```python
from build123d import *

# Parameters (mm, degrees)
BOSS_EXTRUDE1_DEPTH = 1.9
SKETCH2_W           = 2
SKETCH2_H           = 5
BOSS_EXTRUDE2_DEPTH = 0.95


with BuildPart() as part:
    # Sketch1 → Boss-Extrude1 (new body)
    with BuildSketch(Plane(origin=(0, 0, 0), x_dir=(1, 0, 0), z_dir=(0, 1, 0))):
        with BuildLine():
            Line((172.5, 12.5), (0, 12.5))
            Line((0, 12.5), (0, 7.5))
            ThreePointArc((0, 7.5), (1.26826484, 7.391989197), (2.5, 7.071067812))
            ThreePointArc((2.5, 7.071067812), (12.5, 0), (2.5, -7.071067812))
            ThreePointArc((2.5, -7.071067812), (1.26826484, -7.391989197), (0, -7.5))
            Line((0, -7.5), (0, -12.5))
            Line((0, -12.5), (172.5, -12.5))
            ThreePointArc((172.5, -12.5), (182.747548784, 0), (172.5, 12.5))
        make_face()
        with BuildLine():
            ThreePointArc((47.5, -7.071067812), (37.5, 0), (47.5, 7.071067812))
            ThreePointArc((47.5, 7.071067812), (50, 7.5), (52.5, 7.071067812))
            ThreePointArc((52.5, 7.071067812), (55, 7.5), (57.5, 7.071067812))
            ThreePointArc((57.5, 7.071067812), (60, 7.5), (62.5, 7.071067812))
            ThreePointArc((62.5, 7.071067812), (65, 7.5), (67.5, 7.071067812))
            ThreePointArc((67.5, 7.071067812), (70, 7.5), (72.5, 7.071067812))
            ThreePointArc((72.5, 7.071067812), (75, 7.5), (77.5, 7.071067812))
            ThreePointArc((77.5, 7.071067812), (80, 7.5), (82.5, 7.071067812))
            ThreePointArc((82.5, 7.071067812), (85, 7.5), (87.5, 7.071067812))
            ThreePointArc((87.5, 7.071067812), (90, 7.5), (92.5, 7.071067812))
            ThreePointArc((92.5, 7.071067812), (95, 7.5), (97.5, 7.071067812))
            ThreePointArc((97.5, 7.071067812), (100, 7.5), (102.5, 7.071067812))
            ThreePointArc((102.5, 7.071067812), (105, 7.5), (107.5, 7.071067812))
            ThreePointArc((107.5, 7.071067812), (110, 7.5), (112.5, 7.071067812))
            ThreePointArc((112.5, 7.071067812), (122.5, 0), (112.5, -7.071067812))
            ThreePointArc((112.5, -7.071067812), (110, -7.5), (107.5, -7.071067812))
            ThreePointArc((107.5, -7.071067812), (105, -7.5), (102.5, -7.071067812))
            ThreePointArc((102.5, -7.071067812), (100, -7.5), (97.5, -7.071067812))
            ThreePointArc((97.5, -7.071067812), (95, -7.5), (92.5, -7.071067812))
            ThreePointArc((92.5, -7.071067812), (90, -7.5), (87.5, -7.071067812))
            ThreePointArc((87.5, -7.071067812), (85, -7.5), (82.5, -7.071067812))
            ThreePointArc((82.5, -7.071067812), (80, -7.5), (77.5, -7.071067812))
            ThreePointArc((77.5, -7.071067812), (75, -7.5), (72.5, -7.071067812))
            ThreePointArc((72.5, -7.071067812), (70, -7.5), (67.5, -7.071067812))
            ThreePointArc((67.5, -7.071067812), (65, -7.5), (62.5, -7.071067812))
            ThreePointArc((62.5, -7.071067812), (60, -7.5), (57.5, -7.071067812))
            ThreePointArc((57.5, -7.071067812), (55, -7.5), (52.5, -7.071067812))
            ThreePointArc((52.5, -7.071067812), (50, -7.5), (47.5, -7.071067812))
        make_face(mode=Mode.SUBTRACT)
        with BuildLine():
            ThreePointArc((137.5, 7.071067812), (140, 7.5), (142.5, 7.071067812))
            ThreePointArc((142.5, 7.071067812), (145, 7.5), (147.5, 7.071067812))
            ThreePointArc((147.5, 7.071067812), (150, 7.5), (152.5, 7.071067812))
            ThreePointArc((152.5, 7.071067812), (155, 7.5), (157.5, 7.071067812))
            ThreePointArc((157.5, 7.071067812), (160, 7.5), (162.5, 7.071067812))
            ThreePointArc((162.5, 7.071067812), (165, 7.5), (167.5, 7.071067812))
            ThreePointArc((167.5, 7.071067812), (177.5, 0), (167.5, -7.071067812))
            ThreePointArc((167.5, -7.071067812), (165, -7.5), (162.5, -7.071067812))
            ThreePointArc((162.5, -7.071067812), (160, -7.5), (157.5, -7.071067812))
            ThreePointArc((157.5, -7.071067812), (155, -7.5), (152.5, -7.071067812))
            ThreePointArc((152.5, -7.071067812), (150, -7.5), (147.5, -7.071067812))
            ThreePointArc((147.5, -7.071067812), (145, -7.5), (142.5, -7.071067812))
            ThreePointArc((142.5, -7.071067812), (140, -7.5), (137.5, -7.071067812))
            ThreePointArc((137.5, -7.071067812), (127.5, 0), (137.5, 7.071067812))
        make_face(mode=Mode.SUBTRACT)
    extrude(amount=BOSS_EXTRUDE1_DEPTH)

    # Sketch2 → Boss-Extrude2 (add)
    with BuildSketch(Plane(origin=(0, 0, 0), x_dir=(1, 0, 0), z_dir=(0, 1, 0))):
        with Locations((-1, 10)):
            Rectangle(SKETCH2_W, SKETCH2_H)
        with Locations((-1, -10)):
            Rectangle(SKETCH2_W, SKETCH2_H)
    extrude(amount=BOSS_EXTRUDE2_DEPTH)


solid = part.part
```
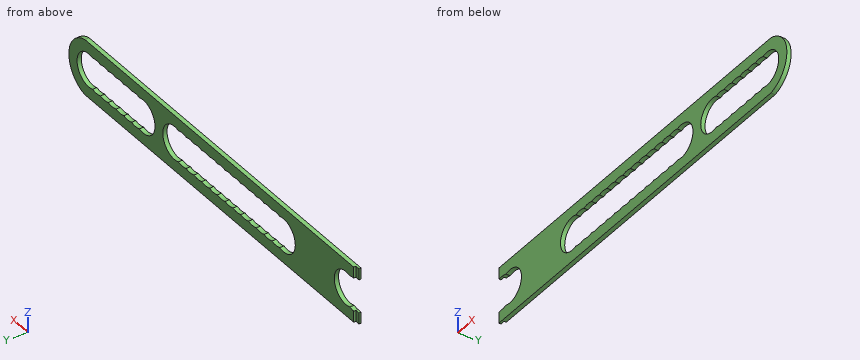
CAD build for the part. Positions are in the model's coordinates, mm. Coordinates: 2 decimals unless noted, no trailing zeros. Order: outer loops, then holes, each group sorted by start corner. A loop starts at its lowest first (then second) coordinate and runs counter-clockwise, first axis right, second up. Notation, with made-up numbers: (-21.75, -20.5) - (37.25, -20.5) arc R15 ccw to (37.25, -2.5) - close; hole circle Ø5 at (78, 38.5). An arc over 180 degrees is marked (long way). Answer in a Markdown table with one row per item.
1. Flat gauge pins, fed straight in: P1, Ø6, axis at x = 88, z = 2.5, coming from the +Y side; P2, Ø1.6, axis at x = -1, z = -9.5, coming from the +Y side. Where does each tip first touch, or does it go through?
Answer:
| item | result |
|---|---|
| P1 | through |
| P2 | y = 0.95 |
2. Slice it at D-D, the plane y = 0.6. Give the number of separate pieces and of enclosed holes in the cut face, then the cut area to 3 significant figures.
Answer:
| item | result |
|---|---|
| separate pieces | 1 |
| enclosed holes | 2 |
| area | 2,460 mm² |
3. Slice it at A-A, the plane z = 0. List the corners of the cut face in (x, y).
Answer:
| item | result |
|---|---|
| outline | (12.5, 0) - (37.5, 0) - (37.5, 1.9) - (12.5, 1.9) - close; (122.5, 0) - (127.5, 0) - (127.5, 1.9) - (122.5, 1.9) - close; (177.5, 0) - (182.75, 0) - (182.75, 1.9) - (177.5, 1.9) - close |
4. Slice it at B-B, the plane x = 115. List the corners of the cut face in (y, z).
Answer:
| item | result |
|---|---|
| outline | (0, -12.5) - (1.9, -12.5) - (1.9, -7.5) - (0, -7.5) - close; (0, 7.5) - (1.9, 7.5) - (1.9, 12.5) - (0, 12.5) - close |
5. Drill centre lines: L1, parallel to Z at x = 135, y = 0.4; L2, parallel to X at y = 1.6, z = 0.75; L3, parallel to X at y = 0.2, z = 1.75. Where is each one in solid material? Low to high. Write a range as from..to.
Answer:
| item | result |
|---|---|
| L1 | -12.5..-7.5, 7.5..12.5 |
| L2 | 12.46..37.54, 122.46..127.54, 177.46..182.73 |
| L3 | 12.29..37.71, 122.29..127.71, 177.29..182.63 |
6. Slice it at C-C, the plane z = 9.5. List the corners of the cut face in (x, y), then the cut area to 3 significant figures.
Answer:
| item | result |
|---|---|
| outline | (-2, 0) - (178.5, 0) - (178.5, 1.9) - (0, 1.9) - (0, 0.95) - (-2, 0.95) - close |
| area | 341 mm² |
